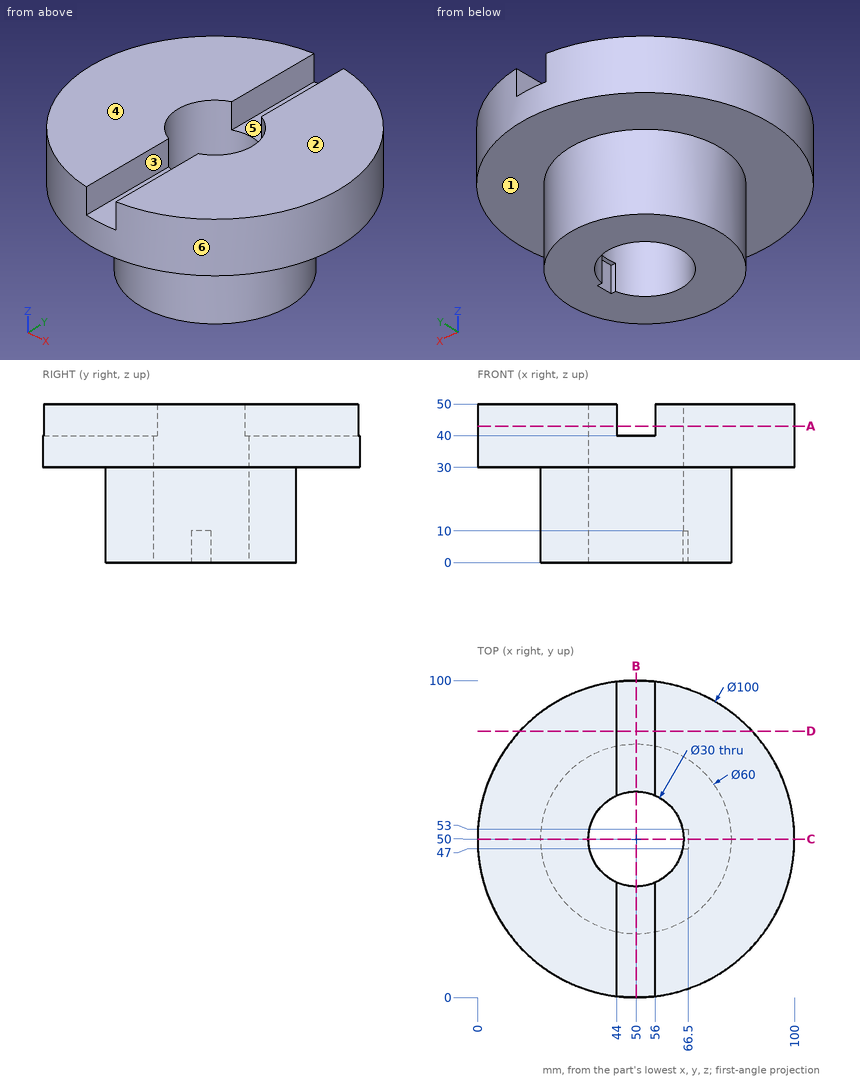
Source: three-view drawing plus pictorial views. Frame: mm from the lowest corner of the part. A direction names the side the tool comes from. Coordinates: 2 decimals unless noted, no trailing zeros. Write each loop counter-clockwise with the first axis right and the second up, starting at its lowest first coordinate (ties: lowest second). Pieces come first, ordered by that corner, then holes. Notation, with made-up numbers: (2.25, 49.5) - (22.25, 49.5) arc R13 ccw to (22.25, 73.5) - close; hole circle Ø1 at (8.25, 34.5). An arc over 180 degrees is marked (long way). Return JSON: item names as keys, results as strings.
Item 1: Reachability of the marked faces 1, 2 and 3 from +Z, -Z, +X, -X, +Y, -Y: full face, straight path, thin tool, end or side. Return the list, or none.
Completed:
{"face 1": "-Z", "face 2": "+Z, +X, -X, +Y, -Y", "face 3": "+Z, +Y, -Y"}
Item 2: Section query B-B (x = 50). Output: boundary loops of the cut face in (y, z).
Completed:
{"outline": "(0, 30) - (20, 30) - (20, 0) - (35, 0) - (35, 40) - (0, 40) - close; (65, 0) - (80, 0) - (80, 30) - (100, 30) - (100, 40) - (65, 40) - close"}
Item 3: Pull-direction query (X, two-part tool) for the marked faces 4, 5 and 6; classes: +X half, -X half, draft (parallel to the pull), parting line (faces both ways), or undercut.
Completed:
{"face 4": "draft", "face 5": "undercut", "face 6": "parting line"}
Item 4: Section query D-D (y = 84). Output: boundary loops of the cut face in (x, z).
Completed:
{"outline": "(13.34, 30) - (86.66, 30) - (86.66, 50) - (56, 50) - (56, 40) - (44, 40) - (44, 50) - (13.34, 50) - close"}
Item 5: Pin query (flat end, axial travel): pin 1 Ø8 at (y, z) = (86, 44.5) entering from -X; pin 2 Ø8 at (y, z) = (9.5, 45.5) entering from +X; pin 3 Ø8 at (y, z) = (46.5, 31) entering from +X; pin 4 Ø6 at (x, z) = (25.5, 33) entering from -Y. Return the tip coordinate at first contact, or that it passes through.
Completed:
{"pin 1": "stops at x = 11.58", "pin 2": "stops at x = 84.17", "pin 3": "stops at x = 100", "pin 4": "stops at y = 4.86"}
Item 6: Line query: L1, parallel to Y at x = 50, z = 20; L2, parallel to X at y = 90, z = 41. Output: solid intervals per line, ascending.
Completed:
{"L1": "y = 20 to 35, 65 to 80", "L2": "x = 20 to 44, 56 to 80"}
Item 7: Section query C-C (y = 50). Output: boundary loops of the cut face in (x, z).
Completed:
{"outline": "(0, 30) - (20, 30) - (20, 0) - (35, 0) - (35, 50) - (0, 50) - close; (65, 10) - (66.5, 10) - (66.5, 0) - (80, 0) - (80, 30) - (100, 30) - (100, 50) - (65, 50) - close"}
Item 8: Section query A-A (z = 43). Output: boundary loops of the cut face in (x, y).
Completed:
{"outline": "(44, 0.36) - (44, 36.25) arc R15 cw to (44, 63.75) - (44, 99.64) arc R50 ccw to start; (56, 0.36) arc R50 ccw to (56, 99.64) - (56, 63.75) arc R15 cw to (56, 36.25) - close"}
